```python
from build123d import *

# Parameters (mm, degrees)
BOSS_EXTRUDE1_DEPTH = 1.6


with BuildPart() as part:
    # Sketch1 → Boss-Extrude1 (new, symmetric)
    with BuildSketch(Plane.XY):
        with BuildLine():
            Line((-82.5, 9.5), (-82.5, -9.5))
            Line((-82.5, -9.5), (-49.642374512, -9.5))
            ThreePointArc((-49.642374512, -9.5), (-39.177078252, -7.253737634), (-28.5, -6.5))
            Line((-28.5, -6.5), (28.5, -6.5))
            ThreePointArc((28.5, -6.5), (39.177078252, -7.253737634), (49.642374512, -9.5))
            Line((49.642374512, -9.5), (82.5, -9.5))
            Line((82.5, -9.5), (82.5, 9.5))
            Line((82.5, 9.5), (49.642374512, 9.5))
            ThreePointArc((49.642374512, 9.5), (39.177078252, 7.253737634), (28.5, 6.5))
            Line((28.5, 6.5), (-28.5, 6.5))
            ThreePointArc((-28.5, 6.5), (-39.177078252, 7.253737634), (-49.642374512, 9.5))
            Line((-49.642374512, 9.5), (-82.5, 9.5))
        make_face()
    extrude(amount=BOSS_EXTRUDE1_DEPTH, both=True)


solid = part.part
```
Read the model definition and answer for the solid it produces. Units are mm, in the model's axes. A direction names the side the tool comes from. Coordinates: 2 decimals unless noted, no trailing zeros. Loops run counter-clockwise (first coordinate to the right, second up) from the corner with the lowest first, then second, coordinate; pieces in that order, holes last.
(1) The part is cut by section A-A (z = -1.1). Determine the outline of the cut face in (x, y), and give its area (3 significant figures).
Solution:
outline: (-82.5, -9.5) - (-49.64, -9.5) arc R76 cw to (-28.5, -6.5) - (28.5, -6.5) arc R76 cw to (49.64, -9.5) - (82.5, -9.5) - (82.5, 9.5) - (49.64, 9.5) arc R76 cw to (28.5, 6.5) - (-28.5, 6.5) arc R76 cw to (-49.64, 9.5) - (-82.5, 9.5) - close
area: 2,620 mm2
(2) The part is cut by section C-C (x = 39). Determine the outline of the cut face in (y, z).
Solution:
outline: (-7.23, -1.6) - (7.23, -1.6) - (7.23, 1.6) - (-7.23, 1.6) - close
(3) The part is cut by section B-B (x = 12.5). Determine the outline of the cut face in (y, z), and give its area (3 significant figures).
Solution:
outline: (-6.5, -1.6) - (6.5, -1.6) - (6.5, 1.6) - (-6.5, 1.6) - close
area: 41.6 mm2
(4) The mould has two halves that part along X. Classify faces 1 (the face through (0, 6.5, 0)), 2 (the face through (-82.5, 0, 0)), 3 (the face through (66, 9.5, 0)): released by +X, released by -X, zero draft, split by the parting line, or undercut.
Solution:
face 1: undercut
face 2: released by -X
face 3: zero draft
(5) A tool of negligible diameter and unlimited length cuts with its end or side. For faces 4 (the face through (82.5, 0, 0)), 5 (the face through (39.326, 7.275, 0.022)), 6 (the face through (0, -6.5, 0)), from which of +Z, -Z, +X, -X, +Y, -Y can it reach the whole face along a straight path? Write none if from no direction.
Solution:
face 4: +Z, -Z, +X, +Y, -Y
face 5: +Z, -Z, +Y
face 6: +Z, -Z, -Y
(6) Consider line 1 along Y through (x, z) = (30, 0.2); line 2 along Y through (x, z) = (44, 1.05). Determine where each line is inside the solid, lowest interval first.
Solution:
line 1: y = -6.51 to 6.51
line 2: y = -8.1 to 8.1
